Read the model definition and answer for the solid it produces. Units are mm, in the model's axes. Face numbers are marked on the shaded views. A direction names the side the tool comes from. Give positions to 0.01 mm unless a question says otherwise; leave off trailing zeros. Order: outer loops, then holes, each group sorted by start corner. A loop starts at its lowest first (then second) coordinate and runs counter-clockwise, first axis right, second up. Notation, with made-up numbers: (-24, -17.5) - (17, -17.5) arc R8 cw to (17, -3.5) - close; hole circle Ø8 at (19.25, 43). An arc over 180 degrees is marked (long way). Write item = value, one per line.
```python
from build123d import *

# Parameters (mm, degrees)
F0_W     = 28
F0_H     = 50
F1_DEPTH = 3
F2_W     = 8
F2_H     = 50
F2_W_2   = 12
F3_DEPTH = 25
F4_W     = 20
F4_H     = 50
F4_W_2   = 8
F5_DEPTH = 3
F7_DEPTH = 67.4


with BuildPart() as f1:
    # F0 (on Top) → F1 (new body)
    with BuildSketch(Plane.XY):
        with Locations((14, 25)):
            Rectangle(F0_W, F0_H)
    extrude(amount=F1_DEPTH)

    # F2 (on face) → F3 (join)
    with BuildSketch(Plane.XY.offset(3)):
        with Locations((4, 25)):
            Rectangle(F2_W, F2_H)
        with Locations((22, 25)):
            Rectangle(F2_W_2, F2_H)
    extrude(amount=F3_DEPTH)

    # F4 (on face) → F5 (join)
    with BuildSketch(Plane.XY.offset(28)):
        with Locations((18, 25)):
            Rectangle(F4_W, F4_H)
        with Locations((4, 25)):
            Rectangle(F4_W_2, F4_H)
    extrude(amount=F5_DEPTH)

    # F6 (on face) → F7 (cut)
    with BuildSketch(Plane.YZ.offset(28)):
        with BuildLine():
            ThreePointArc((26.5, 23), (26.06066, 24.06066), (25, 24.5))
            ThreePointArc((25, 24.5), (23.93934, 21.93934), (26.5, 23))
        make_face()
        with BuildLine():
            ThreePointArc((37.5, 12), (37.06066, 13.06066), (36, 13.5))
            ThreePointArc((36, 13.5), (34.93934, 10.93934), (37.5, 12))
        make_face()
    extrude(amount=-F7_DEPTH, mode=Mode.SUBTRACT)


solid = f1.part
```
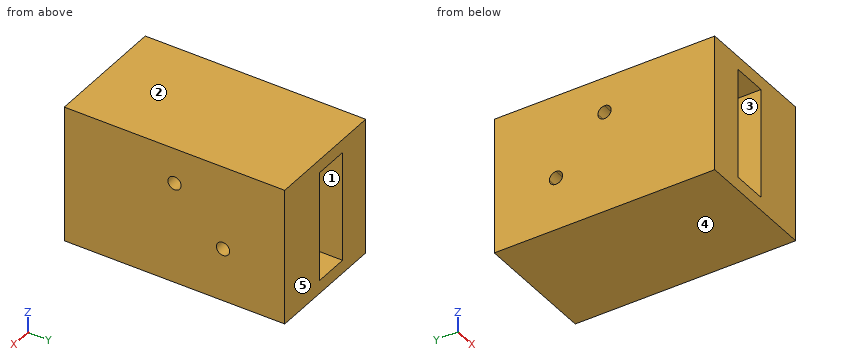
1. Section A-A (y = 12.5) is taken. Determine the outline of the cut face in (x, z), and give its area (3 significant figures).
Recorded:
outline = (0, 0) - (28, 0) - (28, 31) - (0, 31) - close; hole (8, 3) - (16, 3) - (16, 28) - (8, 28) - close
area = 668 mm^2
2. For the marked faces 1 and 2, determine the directions among +Z, -Z, +X, -X, +Y, -Y from which every point of the face is accessible in a straight line to the end or side of a thin tool.
Recorded:
face_1 = +Y, -Y
face_2 = +Z, +X, -X, +Y, -Y
3. Straight lines are drawn through the part: L1, parallel to X at y = 35.5, z = 27; L2, parallel to Y at x = 25.5, z = 23; L3, parallel to Y at x = 20.5, z = 12. For each, find the intervals that lie inside material, in ascending order. Write a range as [from, to].
Recorded:
L1 = [0, 8], [16, 28]
L2 = [0, 23.5], [26.5, 50]
L3 = [0, 34.5], [37.5, 50]
4. Determine the mould class of the marked faces 3, 4 and 5 for opening direction Z: +Z half, -Z half, draft (parallel to the pull), parting line (faces both ways), or undercut.
Recorded:
face_3 = undercut
face_4 = -Z half
face_5 = draft
5. Flat-ended cylindrical pins translate along their axes: pin 1 (4 mm diameter, centred on x = 11, y = 31.5, fed in from -Z); pin 2 (2.5 mm diameter, centred on y = 25, z = 23, fed in from -X). Find the tip coordinate at first contact, or state that the pin passes through.
Recorded:
pin_1 = 0
pin_2 = through
